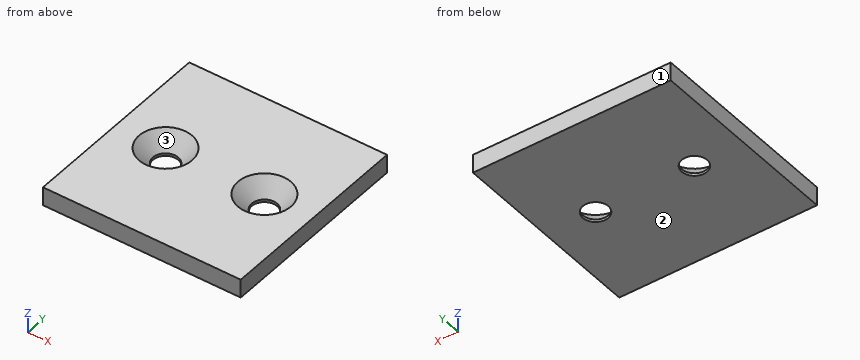
from build123d import *

# Parameters (mm, degrees)
SKETCH1_W           = 50.8
SKETCH1_H           = 50.8
SKETCH1_R           = 3.2639
BOSS_EXTRUDE1_DEPTH = 2.3876
CUT_EXTRUDE1_START  = -4.0894
SKETCH2_R           = 3.2639
CUT_EXTRUDE1_DEPTH  = 5.0894
CUT_EXTRUDE1_TAPER  = -41


with BuildPart() as part:
    # Sketch1 → Boss-Extrude1 (new body, symmetric)
    with BuildSketch(Plane.XY):
        with Locations((25.4, 25.4)):
            Rectangle(SKETCH1_W, SKETCH1_H)
        with Locations((12.7, 25.4)):
            Circle(SKETCH1_R, mode=Mode.SUBTRACT)
        with Locations((38.1, 25.4)):
            Circle(SKETCH1_R, mode=Mode.SUBTRACT)
    extrude(amount=BOSS_EXTRUDE1_DEPTH, both=True)

    # Sketch2 → Cut-Extrude1 (cut, through all)
    with BuildSketch(Plane.XY.offset(2.3876).offset(CUT_EXTRUDE1_START)):
        with Locations((12.7, 25.4)):
            Circle(SKETCH2_R)
        with Locations((38.1, 25.4)):
            Circle(SKETCH2_R)
    extrude(amount=CUT_EXTRUDE1_DEPTH, taper=CUT_EXTRUDE1_TAPER, mode=Mode.SUBTRACT)


solid = part.part
The model under review builds one solid part; all positions refer to its coordinate system, in mm. Face numbers are marked on the shaded views. Round coordinates to 2 decimals unless told otherwise and drop trailing zeros. Write each loop counter-clockwise with the first axis right and the second up, starting at its lowest first coordinate (ties: lowest second). Pieces come first, ordered by that corner, then holes. Notation, with made-up numbers: (7, 43.25) -> (55, 43.25) arc R23 cw to (55, 78.25) -> close; hole circle Ø3 at (59, 66.5). An arc over 180 degrees is marked (long way). Answer as a JSON object with one key per item and string values.
1. We need section A-A on x = 38.1. State the section outline as (y, z) points, and give its area (3 significant figures).
Results found:
{"outline": "(0, -2.39) -> (22.14, -2.39) -> (22.14, -1.7) -> (18.58, 2.39) -> (0, 2.39) -> close; (28.66, -2.39) -> (50.8, -2.39) -> (50.8, 2.39) -> (32.22, 2.39) -> (28.66, -1.7) -> close", "area": "197 mm^2"}
2. We need section C-C on z = -1.05. State the section outline as (x, y) points, and give its area (3 significant figures).
Results found:
{"outline": "(0, 0) -> (50.8, 0) -> (50.8, 50.8) -> (0, 50.8) -> close; hole circle Ø7.66 at (12.7, 25.4); hole circle Ø7.66 at (38.1, 25.4)", "area": "2,490 mm^2"}
3. To check wall thickness, follow line 1 along Y through (x, z) = (12.7, -2.05); line 2 along X through (y, z) = (22.5, 0.45); line 3 along Y through (x, z) = (11.5, -0.55). State the ranges of each line that lie inside material, in increasing order.
Results found:
{"line 1": "y = 0 to 22.14, 28.66 to 50.8", "line 2": "x = 0 to 8.46, 16.94 to 33.86, 42.34 to 50.8", "line 3": "y = 0 to 21.31, 29.49 to 50.8"}
4. We need section B-B on y = 25.4. State how many separate pieces and enclosed holes the cut face has, and give its area (3 significant figures).
Results found:
{"separate pieces": "3", "enclosed holes": "0", "area": "151 mm^2"}
5. The part is to be moulded in two halves that separate along Y. For the marked faces 1, 2 and 3, say which applies: pulls with the +Y half, pulls with the -Y half, needs draft (parallel to the pull), parting line crosses it, or undercut.
Results found:
{"face 1": "pulls with the +Y half", "face 2": "needs draft", "face 3": "undercut"}
